The drawing under review shows one solid part. Ordinate dimensions are in mm from its lowest x, y, z. A direction names the side the tool comes from. Round coordinates to 2 decimals unless told otherwise and drop trailing zeros. Write each loop counter-clockwise with the first axis right and the second up, starting at its lowest first coordinate (ties: lowest second). Pieces come first, ordered by that corner, then holes. Notation, with made-up numbers: (-13, 19.25) -> (12, 19.25) arc R23 cw to (12, 46.25) -> close; hole circle Ø1 at (-16.5, 9). An arc over 180 degrees is marked (long way). Write item = value, one per line. Start each with the question number.
Item 1: Add section D-D, the plane x = 10. State the section outline as (y, z) points (1 decimal).
Item 2: To check wall thickness, follow L1, parallel to Y at x = 38, z = 27 (1 decimal); L2, parallel to X at y = 43, z = 4 (1 decimal); L3, parallel to Z at x = 6, y = 43. State the ranges of each line that lie inside material, in increasing order.
Item 3: Machinability: for the marked faces 1, 2 and 3, which of the approach directions +Z, -Z, +X, -X, +Y, -Y give a long, thin tool a straight path to every point of the face, cutting with its end or side? Answer none if there is none.
Item 4: Add section B-B, the plane z = 52.5. State the section outline as (x, y) points (1 decimal).
Item 5: Mouldability with a two-part tool opening along Y and no side actions: class the marked faces 4, 5 and 6 as released by +Y, released by -Y, zero draft, split by the parting line, or undercut.
Item 6: For pin 1 Ø1 at (x, y) = (71.5, 14.5) entering from +Z; pin 2 Ø4 at (y, z) = (70.5, 30.5) entering from +X; pin 3 Ø4 at (y, z) = (6, 12.5) entering from +X; pin 4 Ø18 at (x, z) = (28.575, 44.45) entering from -Y, all flat-tipped, find the tip position at first contact; note any pin that passes through.
Item 7: Add section C-C, the plane x = 78. State the section outline as (y, z) points (1 decimal).
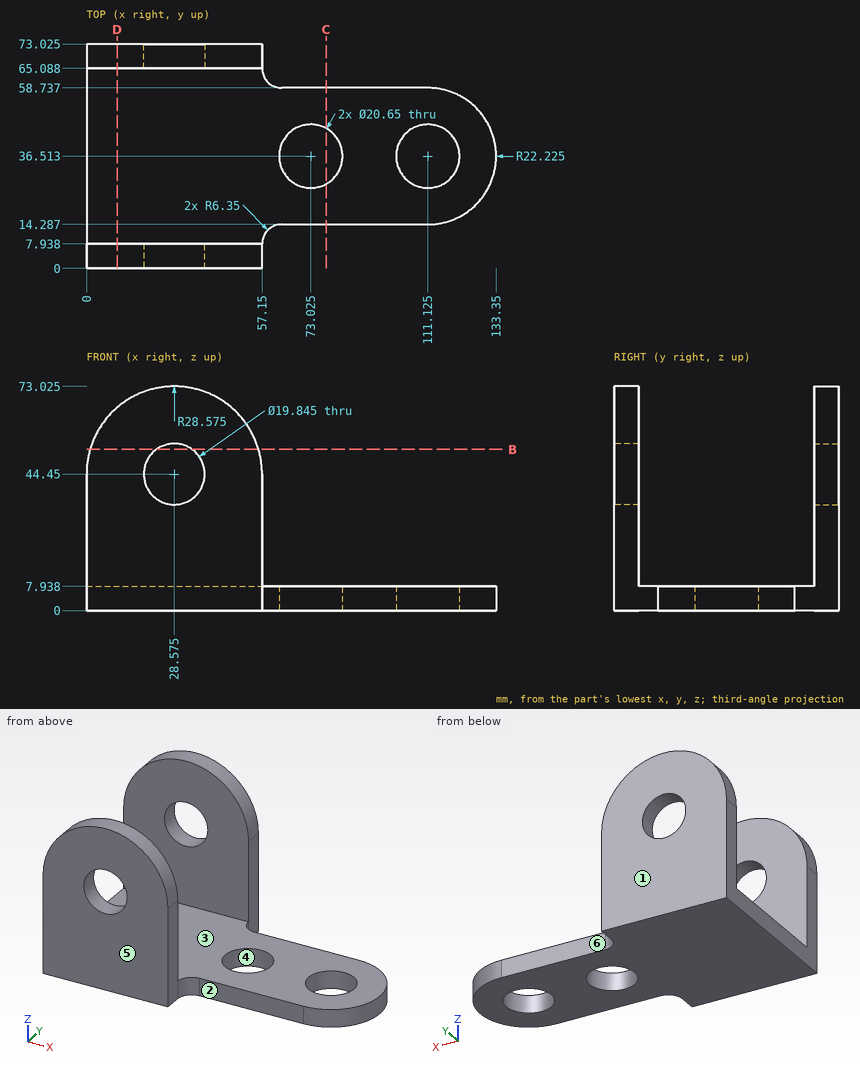
Result set:
q1.outline = (0, 0) -> (73, 0) -> (73, 66.2) -> (65.1, 66.2) -> (65.1, 7.9) -> (7.9, 7.9) -> (7.9, 66.2) -> (0, 66.2) -> close
q2.L1 = 0 to 7.9, 65.1 to 73
q2.L2 = 0 to 65, 81.1 to 103.1, 119.2 to 132.4
q2.L3 = 0 to 7.94
q3.face_1 = +Z, -Z, +X, -X, +Y
q3.face_2 = +Z, -Z, +X, -Y
q3.face_3 = +Z, +X, -X
q4.outline = (1.2, 0) -> (22.8, 0) -> (22.8, 7.9) -> (1.2, 7.9) -> close; (1.2, 65.1) -> (22.8, 65.1) -> (22.8, 73) -> (1.2, 73) -> close; (34.4, 0) -> (56, 0) -> (56, 7.9) -> (34.4, 7.9) -> close; (34.4, 65.1) -> (56, 65.1) -> (56, 73) -> (34.4, 73) -> close
q5.face_4 = undercut
q5.face_5 = released by -Y
q5.face_6 = released by +Y
q6.pin_1 = 7.94
q6.pin_2 = 57.15
q6.pin_3 = 57.15
q6.pin_4 = through
q7.outline = (14.3, 0) -> (27.5, 0) -> (27.5, 7.9) -> (14.3, 7.9) -> close; (45.6, 0) -> (58.7, 0) -> (58.7, 7.9) -> (45.6, 7.9) -> close
